from build123d import *

# Parameters (mm, degrees)
BOSS_EXTRUDE1_DEPTH = 44.45
SKETCH2_R           = 3.429
CUT_EXTRUDE1_DEPTH  = 44.45
SKETCH3_R           = 3.429
CUT_EXTRUDE2_DEPTH  = 44.45
CUT_EXTRUDE3_DEPTH  = 5.588
CUT_EXTRUDE4_DEPTH  = 5.588
BOSS_EXTRUDE2_DEPTH = 3.175
FILLET1_R           = 2.54


with BuildPart() as part:
    # Sketch1 → Boss-Extrude1 (new body)
    with BuildSketch(Plane.XY):
        Polygon((0, 0), (63.5, 0), (63.5, 10.16), (6.788694961, 10.16), (46.889643324, 50.260948363), (39.705438427, 57.44515326), (-5.195842178, 12.543872654), align=None)
    extrude(amount=BOSS_EXTRUDE1_DEPTH)

    # Sketch2 → Cut-Extrude1 (cut)
    with BuildSketch(Plane(origin=(0, 10.16, 0), x_dir=(1, 0, 0), z_dir=(0, 1, 0))):
        with Locations((53.34, -34.925)):
            Circle(SKETCH2_R)
        with Locations((53.34, -9.525)):
            Circle(SKETCH2_R)
        with Locations((27.94, -9.525)):
            Circle(SKETCH2_R)
        with Locations((27.94, -34.925)):
            Circle(SKETCH2_R)
    extrude(amount=-CUT_EXTRUDE1_DEPTH, mode=Mode.SUBTRACT)

    # Sketch3 → Cut-Extrude2 (cut)
    with BuildSketch(Plane(origin=(-1.685652519, 1.685652519, 0), x_dir=(0, 0, -1), z_dir=(0.707106781, -0.707106781, 0))):
        with Locations((-9.525, 33.135842178)):
            Circle(SKETCH3_R)
        with Locations((-9.525, 58.535842178)):
            Circle(SKETCH3_R)
        with Locations((-34.925, 58.535842178)):
            Circle(SKETCH3_R)
        with Locations((-34.925, 33.135842178)):
            Circle(SKETCH3_R)
    extrude(amount=-CUT_EXTRUDE2_DEPTH, mode=Mode.SUBTRACT)

    # Sketch4 → Cut-Extrude3 (cut)
    with BuildSketch(Plane(origin=(0, 10.16, 0), x_dir=(1, 0, 0), z_dir=(0, 1, 0))):
        Polygon((22.225, -31.625443212), (22.225, -38.224556788), (27.94, -41.524113577), (33.655, -38.224556788), (33.655, -31.625443212), (27.94, -28.325886423), align=None)
        Polygon((47.625, -31.625443212), (47.625, -38.224556788), (53.34, -41.524113577), (59.055, -38.224556788), (59.055, -31.625443212), (53.34, -28.325886423), align=None)
        Polygon((22.225, -6.225443212), (22.225, -12.824556788), (27.94, -16.124113577), (33.655, -12.824556788), (33.655, -6.225443212), (27.94, -2.925886423), align=None)
        Polygon((47.625, -6.225443212), (47.625, -12.824556788), (53.34, -16.124113577), (59.055, -12.824556788), (59.055, -6.225443212), (53.34, -2.925886423), align=None)
    extrude(amount=-CUT_EXTRUDE3_DEPTH, mode=Mode.SUBTRACT)

    # Sketch5 → Cut-Extrude4 (cut)
    with BuildSketch(Plane(origin=(-1.685652519, 1.685652519, 0), x_dir=(0, 0, -1), z_dir=(0.707106781, -0.707106781, 0))):
        Polygon((-2.925886423, 58.535842178), (-6.225443212, 64.250842178), (-12.824556788, 64.250842178), (-16.124113577, 58.535842178), (-12.824556788, 52.820842178), (-6.225443212, 52.820842178), align=None)
        Polygon((-28.325886423, 58.535842178), (-31.625443212, 64.250842178), (-38.224556788, 64.250842178), (-41.524113577, 58.535842178), (-38.224556788, 52.820842178), (-31.625443212, 52.820842178), align=None)
        Polygon((-2.925886423, 33.135842178), (-6.225443212, 38.850842178), (-12.824556788, 38.850842178), (-16.124113577, 33.135842178), (-12.824556788, 27.420842178), (-6.225443212, 27.420842178), align=None)
        Polygon((-28.325886423, 33.135842178), (-31.625443212, 38.850842178), (-38.224556788, 38.850842178), (-41.524113577, 33.135842178), (-38.224556788, 27.420842178), (-31.625443212, 27.420842178), align=None)
    extrude(amount=-CUT_EXTRUDE4_DEPTH, mode=Mode.SUBTRACT)

    # Sketch6 → Boss-Extrude2 (add, symmetric)
    with BuildSketch(Plane.XY.offset(22.225)):
        Polygon((6.788694961, 10.16), (33.729463324, 37.100768363), (44.888694961, 10.16), align=None)
    extrude(amount=BOSS_EXTRUDE2_DEPTH, both=True)

    # Fillet1
    fillet1_edges = [part.edges().sort_by_distance(p)[0] for p in [
        (-5.195842178, 12.543872654, 22.225),
        (39.705438427, 57.44515326, 22.225),
        (46.889643324, 50.260948363, 22.225),
        (6.788694961, 10.16, 34.925),
        (63.5, 10.16, 22.225),
        (63.5, 0, 22.225),
        (0, 0, 22.225),
        (6.788694961, 10.16, 9.525),
        (25.838694961, 10.16, 19.05),
        (44.888694961, 10.16, 22.225),
        (20.259079143, 23.630384182, 19.05),
        (33.729463324, 37.100768363, 22.225),
        (25.838694961, 10.16, 25.4),
        (20.259079143, 23.630384182, 25.4),
    ]]
    fillet(fillet1_edges, radius=FILLET1_R)


solid = part.part
The listing builds one solid part. Answer for the finished solid, in the listing's coordinates (mm). A direction names the side the tool comes from. Round coordinates to 2 decimals unless told otherwise and drop trailing zeros. Write each loop counter-clockwise with the first axis right and the second up, starting at its lowest first coordinate (ties: lowest second). Pieces come first, ordered by that corner, then holes. Notation, with made-up numbers: M 53.25,-3 L 76.25,-3 A15 cw 76.25,15 Z; hole C -7,77.25 d6. An arc over 180 degrees is marked long. Write each question's results on one line, items separated by ' | '. Start each with the question number.
Item 1: The mould has two halves that part along Y. Classify faces 1 (the flat face through (15.76, 23.02, 9.57)), 2 (the flat face through (17.748, 25.015, 4.599)), 3 (the cylindrical face through (25.41, 2.32, 32.61)), 4 (the flat face through (50.7, 4.572, 12.4)): +Y half, -Y half, draft (parallel to the pull), parting line (faces both ways), or undercut.
Item 2: Straight lines are drawn through the part: probe 1 along Z at (x, y) = (53, 3); probe 2 along Z at (x, y) = (27, 1); probe 3 along Y at (x, z) = (14.5, 36). For each, find the intervals that lie inside material, in ascending order.
Item 3: Which of the six approach directions +Z, -Z, +X, -X, +Y, -Y give full straight-line access (tool end or side, diameter ignored) to faces 5 (the flat face through (50.523, 7.405, 4.553)), 6 (the flat face through (30.84, 7.41, 30)), 7 (the cylindrical face through (23.71, 26.05, 26.16)), 8 (the flat face through (39.24, 23.8, 22.27))?
Item 4: Find section A-A on y = 8.5. Write down the section's boundary in (x, z) (3 decimals).
Item 5: Given pin 1 Ø6 at (x, z) = (55.5, 27.5) entering from +Y; pin 2 Ø1 at (y, z) = (31.5, 39) entering from -X; pin 3 Ø1.5 at (x, z) = (15.5, 19) entering from +Y, each flat-ended and moving along its own axis, determine where each tip first touches the part or whether it passes through.
Answer block:
1) face 1: undercut | face 2: undercut | face 3: draft | face 4: +Y half
2) probe 1: z = 0 to 6.11, 12.94 to 31.51, 38.34 to 44.45 | probe 2: z = 0 to 6.23, 12.82 to 31.63, 38.22 to 44.45 | probe 3: y = 0 to 10.16, 17.87 to 24.28, 25.77 to 27.76
3) face 5: +Y | face 6: none | face 7: +Z, +X | face 8: +Z, -Z, +X
4) outline: M -3.521,0 L 63.343,0 L 63.343,44.45 L -3.521,44.45 Z; hole M 22.225,6.225 L 27.94,2.926 L 33.655,6.225 L 33.655,12.825 L 27.94,16.124 L 22.225,12.825 Z; hole M 22.225,31.625 L 27.94,28.326 L 33.655,31.625 L 33.655,38.225 L 27.94,41.524 L 22.225,38.225 Z; hole M 47.625,6.225 L 53.34,2.926 L 59.055,6.225 L 59.055,12.825 L 53.34,16.124 L 47.625,12.825 Z; hole M 47.625,31.625 L 53.34,28.326 L 59.055,31.625 L 59.055,38.225 L 53.34,41.524 L 47.625,38.225 Z
5) pin 1: stops at y = 10.16 | pin 2: stops at x = 13.26 | pin 3: stops at y = 33.99
